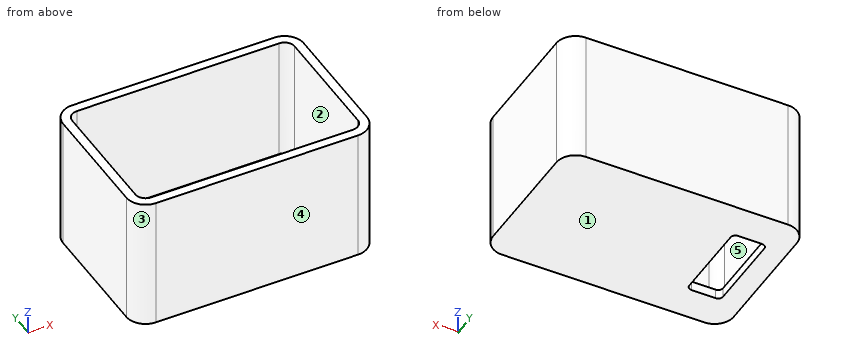
from build123d import *

# Parameters (mm, degrees)
BOSS_EXTRUDE1_DEPTH = 28
BOSS_EXTRUDE2_DEPTH = 2


with BuildPart() as part:
    # Sketch1 → Boss-Extrude1 (new body)
    with BuildSketch(Plane.XY):
        with BuildLine():
            ThreePointArc((-25, 12.25), (-23.828427125, 15.078427125), (-21, 16.25))
            Line((-21, 16.25), (21, 16.25))
            ThreePointArc((21, 16.25), (23.828427125, 15.078427125), (25, 12.25))
            Line((25, 12.25), (25, -12.25))
            ThreePointArc((25, -12.25), (23.828427125, -15.078427125), (21, -16.25))
            Line((21, -16.25), (-21, -16.25))
            ThreePointArc((-21, -16.25), (-23.828427125, -15.078427125), (-25, -12.25))
            Line((-25, -12.25), (-25, 12.25))
        make_face()
        with BuildLine():
            Line((-23.1, -12.25), (-23.1, 12.25))
            ThreePointArc((-23.1, 12.25), (-22.48492424, 13.73492424), (-21, 14.35))
            Line((-21, 14.35), (21, 14.35))
            ThreePointArc((21, 14.35), (22.48492424, 13.73492424), (23.1, 12.25))
            Line((23.1, 12.25), (23.1, -12.25))
            ThreePointArc((23.1, -12.25), (22.48492424, -13.73492424), (21, -14.35))
            Line((21, -14.35), (-21, -14.35))
            ThreePointArc((-21, -14.35), (-22.48492424, -13.73492424), (-23.1, -12.25))
        make_face(mode=Mode.SUBTRACT)
    extrude(amount=BOSS_EXTRUDE1_DEPTH)

    # Sketch1_3 → Boss-Extrude2 (add)
    with BuildSketch(Plane.XY):
        with BuildLine():
            ThreePointArc((-23.1, 12.25), (-22.48492424, 13.73492424), (-21, 14.35))
            Line((-21, 14.35), (21, 14.35))
            ThreePointArc((21, 14.35), (22.48492424, 13.73492424), (23.1, 12.25))
            Line((23.1, 12.25), (23.1, -12.25))
            ThreePointArc((23.1, -12.25), (22.48492424, -13.73492424), (21, -14.35))
            Line((21, -14.35), (-21, -14.35))
            ThreePointArc((-21, -14.35), (-22.48492424, -13.73492424), (-23.1, -12.25))
            Line((-23.1, -12.25), (-23.1, 12.25))
        make_face()
        with BuildLine():
            Line((-20.5, -8), (-20.5, 8))
            ThreePointArc((-20.5, 8), (-20.207106781, 8.707106781), (-19.5, 9))
            Line((-19.5, 9), (-14.5, 9))
            ThreePointArc((-14.5, 9), (-13.792893219, 8.707106781), (-13.5, 8))
            Line((-13.5, 8), (-13.5, -8))
            ThreePointArc((-13.5, -8), (-13.792893219, -8.707106781), (-14.5, -9))
            Line((-14.5, -9), (-19.5, -9))
            ThreePointArc((-19.5, -9), (-20.207106781, -8.707106781), (-20.5, -8))
        make_face(mode=Mode.SUBTRACT)
    extrude(amount=BOSS_EXTRUDE2_DEPTH)


solid = part.part
Could you check a few things on this model? Use its own coordinates, in mm. Face numbers are marked on the shaded views. A direction names the side the tool comes from. Give positions to 0.01 mm unless a question says otherwise; leave off trailing zeros. Order: outer loops, then holes, each group sorted by start corner. A loop starts at its lowest first (then second) coordinate and runs counter-clockwise, first axis right, second up. Notation, with made-up numbers: M 35.25,-18 L 81.25,-18 A28 cw 81.25,6 Z; hole C -35.75,8.5 d4. An arc over 180 degrees is marked long. One line per question, with ' | ' between items.
1. For the marked faces 4 and 5, which set-ups out of +Z, -Z, +X, -X, +Y, -Y let a thin tool reach every point of the face, with its end or its side?
Results:
face 4: +Z, -Z, +X, -X, -Y | face 5: +Z
2. I'm going to push a flat-ended pin straight in: pin 1 (10 mm diameter, centred on x = -8.5, y = -10.5, fed in from +Z). Where does the tip first touch, or does it pass through?
Results:
pin 1: z = 28
3. I want a section at D-D (x = 17). List the corners of the cut face in (y, z) for me.
Results:
outline: M -16.25,0 L 16.25,0 L 16.25,28 L 14.35,28 L 14.35,2 L -14.35,2 L -14.35,28 L -16.25,28 Z
4. I want a section at C-C (y = -4.5). List the corners of the cut face in (x, z) for me.
Results:
outline: M -25,0 L -20.5,0 L -20.5,2 L -23.1,2 L -23.1,28 L -25,28 Z; M -13.5,0 L 25,0 L 25,28 L 23.1,28 L 23.1,2 L -13.5,2 Z
5. I want a section at A-A (x = -18). List the corners of the cut face in (y, z) for me, and give its area (3 significant figures).
Results:
outline: M -16.25,0 L -9,0 L -9,2 L -14.35,2 L -14.35,28 L -16.25,28 Z; M 9,0 L 16.25,0 L 16.25,28 L 14.35,28 L 14.35,2 L 9,2 Z | area: 128 mm²
6. If I drill on line 1 (X direction, y = 6, z = 22); line 2 (Y direction, x = -12, z = 13.25); line 3 (Z direction, x = 10.5, y = 14), over which ranges is the centre line in solid material (lowest first)?
Results:
line 1: -25 to -23.1, 23.1 to 25 | line 2: -16.25 to -14.35, 14.35 to 16.25 | line 3: 0 to 2
7. We'd pull the mould along Y, two halves only. Please class the marked faces 1, 2 and 3: +Y half, -Y half, draft (parallel to the pull), parting line (faces both ways), or undercut.
Results:
face 1: draft | face 2: undercut | face 3: -Y half
8. I want a section at B-B (z = 18.75). List the corners of the cut face in (x, y) for me, and give its area (3 significant figures).
Results:
outline: M -25,-12.25 A4 ccw -21,-16.25 L 21,-16.25 A4 ccw 25,-12.25 L 25,12.25 A4 ccw 21,16.25 L -21,16.25 A4 ccw -25,12.25 Z; hole M -23.1,-12.25 A2.1 ccw -21,-14.35 L 21,-14.35 A2.1 ccw 23.1,-12.25 L 23.1,12.25 A2.1 ccw 21,14.35 L -21,14.35 A2.1 ccw -23.1,12.25 Z | area: 289 mm²
